from build123d import *

# Parameters (mm, degrees)
F1_DEPTH    = 4
F2_T1_DEPTH = 43.5711374279
F2_T3_DEPTH = 43.5711374279
F2_T5_DEPTH = 43.5711374279
F2_T7_DEPTH = 43.5711374279
F2_T9_DEPTH = 43.5711374279


# Not quite as in the source:
# - a fillet or chamfer that OpenCascade refuses, or shapes differently, is made with other operations: its cross-section is extruded or revolved along the edge and cut away or added


with BuildPart() as f1:
    # F0 (on Top) → F1 (new body)
    with BuildSketch(Plane.XY):
        Polygon((-9.53812, 16.5205084487), (0, 0), (9.53812, 16.5205084487), align=None)
        Polygon((-19.07624, 0), (0, 0), (-9.53812, 16.5205084487), align=None)
        Polygon((-9.53812, -16.5205084487), (0, 0), (-19.07624, 0), align=None)
        Polygon((9.53812, -16.5205084487), (0, 0), (-9.53812, -16.5205084487), align=None)
        Polygon((19.07624, 0), (0, 0), (9.53812, -16.5205084487), align=None)
        Polygon((9.53812, 16.5205084487), (0, 0), (19.07624, 0), align=None)
    extrude(amount=F1_DEPTH)

    # F2: fillet of radius 5 on 6 edges, made by hand

    # F2_s2 → F2_t1 (cut)
    with BuildSketch(Plane.YZ.offset(-21.7855687139)):
        with BuildLine():
            ThreePointArc((16.5205084487, 0), (14.7838066233, 2.8729833462), (11.6215289631, 4))
            Line((11.6215289631, 4), (16.5205084487, 4))
            Line((16.5205084487, 4), (16.5205084487, 0))
        make_face()
        with BuildLine():
            ThreePointArc((-16.5205084487, 0), (-14.7838066233, 2.8729833462), (-11.6215289631, 4))
            Line((-11.6215289631, 4), (-16.5205084487, 4))
            Line((-16.5205084487, 4), (-16.5205084487, 0))
        make_face()
    extrude(amount=F2_T1_DEPTH, mode=Mode.SUBTRACT)

    # F2_s4 → F2_t3 (cut)
    with BuildSketch(Plane(origin=(10.892784357, 18.8668559422, 0), x_dir=(0, 0, 1), z_dir=(-0.5, -0.8660254038, 0))):
        with BuildLine():
            ThreePointArc((0, 16.5205084487), (2.8729833462, 14.7838066233), (4, 11.6215289631))
            Line((4, 11.6215289631), (4, 16.5205084487))
            Line((4, 16.5205084487), (0, 16.5205084487))
        make_face()
    extrude(amount=F2_T3_DEPTH, mode=Mode.SUBTRACT)

    # F2_s6 → F2_t5 (cut)
    with BuildSketch(Plane(origin=(-10.892784357, 18.8668559422, 0), x_dir=(0, 0, 1), z_dir=(0.5, -0.8660254038, 0))):
        with BuildLine():
            ThreePointArc((0, 16.5205084487), (2.8729833462, 14.7838066233), (4, 11.6215289631))
            Line((4, 11.6215289631), (4, 16.5205084487))
            Line((4, 16.5205084487), (0, 16.5205084487))
        make_face()
    extrude(amount=F2_T5_DEPTH, mode=Mode.SUBTRACT)

    # F2_s8 → F2_t7 (cut)
    with BuildSketch(Plane(origin=(10.892784357, -18.8668559422, 0), x_dir=(0, 0, 1), z_dir=(-0.5, 0.8660254038, 0))):
        with BuildLine():
            ThreePointArc((0, 16.5205084487), (2.8729833462, 14.7838066233), (4, 11.6215289631))
            Line((4, 11.6215289631), (4, 16.5205084487))
            Line((4, 16.5205084487), (0, 16.5205084487))
        make_face()
    extrude(amount=F2_T7_DEPTH, mode=Mode.SUBTRACT)

    # F2_s10 → F2_t9 (cut)
    with BuildSketch(Plane(origin=(-10.892784357, -18.8668559422, 0), x_dir=(0, 0, 1), z_dir=(0.5, 0.8660254038, 0))):
        with BuildLine():
            ThreePointArc((0, 16.5205084487), (2.8729833462, 14.7838066233), (4, 11.6215289631))
            Line((4, 11.6215289631), (4, 16.5205084487))
            Line((4, 16.5205084487), (0, 16.5205084487))
        make_face()
    extrude(amount=F2_T9_DEPTH, mode=Mode.SUBTRACT)


solid = f1.part
Part model, mm, in its own coordinate system. Give positions to 0.01 mm unless a question says otherwise; leave off trailing zeros. Write each loop counter-clockwise with the first axis right and the second up, starting at its lowest first coordinate (ties: lowest second). Pieces come first, ordered by that corner, then holes.
1) Cut at A-A on z = 1.3. Write the cut outline in (x, y).
Resolved:
outline: (-18.55, 0) - (-9.27, -16.06) - (9.27, -16.06) - (18.55, 0) - (9.27, 16.06) - (-9.27, 16.06) - close
2) Probe L1, parallel to Y at x = -6.5, z = 3.55; L2, parallel to X at y = -7, z = 0.65; L3, parallel to Y at x = 4, z = 1.3. List the from-to ranges inside material, lowest first.
Resolved:
L1: y = -13.69 to 13.69
L2: x = -14.83 to 14.83
L3: y = -16.06 to 16.06
3) Pin check, flat tip, straight feed: pin 1 (1.5 mm diameter, centred on x = 13, z = 2, fed in from -Y). Stop position of the tip, or through.
Resolved:
pin 1: stops at y = -10.37
4) Cut at B-B on x = -6. Write the cut outline in (y, z), then the cut area to 3 significant figures.
Resolved:
outline: (-16.52, 0) - (16.52, 0) arc R5 ccw to (11.62, 4) - (-11.62, 4) arc R5 ccw to start
area: 122 mm2
5) Cut at C-C on z = 3.55. Write the cut outline in (x, y), then the cut area to 3 significant figures.
Resolved:
outline: (-15.81, 0) - (-7.91, -13.69) - (7.91, -13.69) - (15.81, 0) - (7.91, 13.69) - (-7.91, 13.69) - close
area: 650 mm2
